Check sheet for the drawn part. Datum: minimum x, y, z corner. Units: mm. Coordinates: 2 decimals unless noted, no trailing zeros. Write each loop counter-clockwise with the first axis right and the second up, starting at its lowest first coordinate (ties: lowest second). Pieces come first, ordered by that corner, then holes. Notation, with made-up numbers: (28, 33) -> (38, 33) arc R31 ccw to (38, 57) -> close; hole circle Ø8 at (37.25, -21). An arc over 180 degrees is marked (long way). Answer in a Markdown table with one row per item.
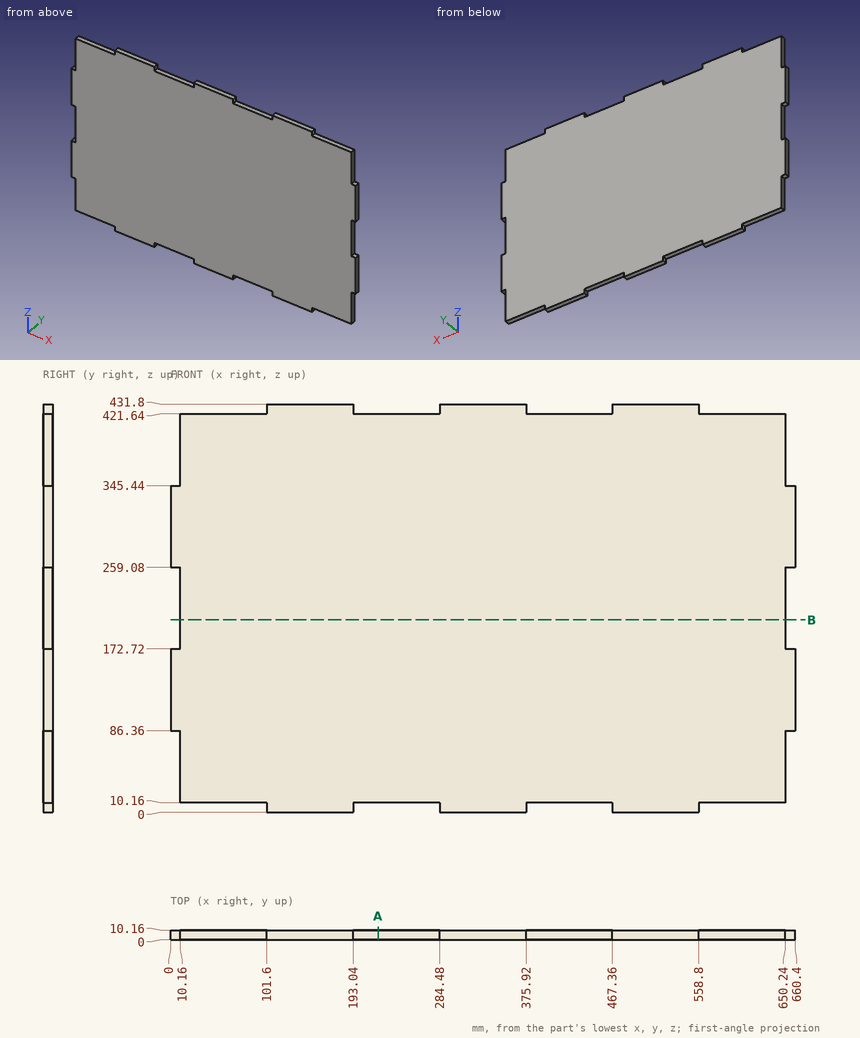
1. Sectioned sample at B-B, the plane z = 203.5. Record the cut outline in (x, y), and give its area (3 significant figures).
Findings below:
| item | result |
|---|---|
| outline | (10.16, 0) -> (650.24, 0) -> (650.24, 10.16) -> (10.16, 10.16) -> close |
| area | 6,500 mm² |
2. Go/stop test with flat-tipped pins: pin 1 (1 mm diameter, centred on x = 471, z = 105, fed in from -Y); pin 2 (5 mm diameter, centred on y = 2.5, z = 365.5, fed in from +X); pin 3 (3 mm diameter, centred on x = 219.5, y = 5.5, fed in from +Z); pin 4 (1 mm diameter, centred on x = 583.5, y = 9, fed in from -Z). Record where each tip stops, or that it passes through.
Findings below:
| item | result |
|---|---|
| pin 1 | stops at y = 0 |
| pin 2 | stops at x = 650.24 |
| pin 3 | stops at z = 421.64 |
| pin 4 | stops at z = 10.16 |
3. Sectioned sample at A-A, the plane x = 219.5. Record the cut outline in (y, z).
Findings below:
| item | result |
|---|---|
| outline | (0, 10.16) -> (10.16, 10.16) -> (10.16, 421.64) -> (0, 421.64) -> close |
4. Material ranges on probe 1 along X at (y, z) = (1.5, 196.5); probe 2 along Z at (x, y) = (567.5, 5.25), recorded low to high. Write a range as from..to.
Findings below:
| item | result |
|---|---|
| probe 1 | x = 10.16..650.24 |
| probe 2 | z = 10.16..421.64 |
